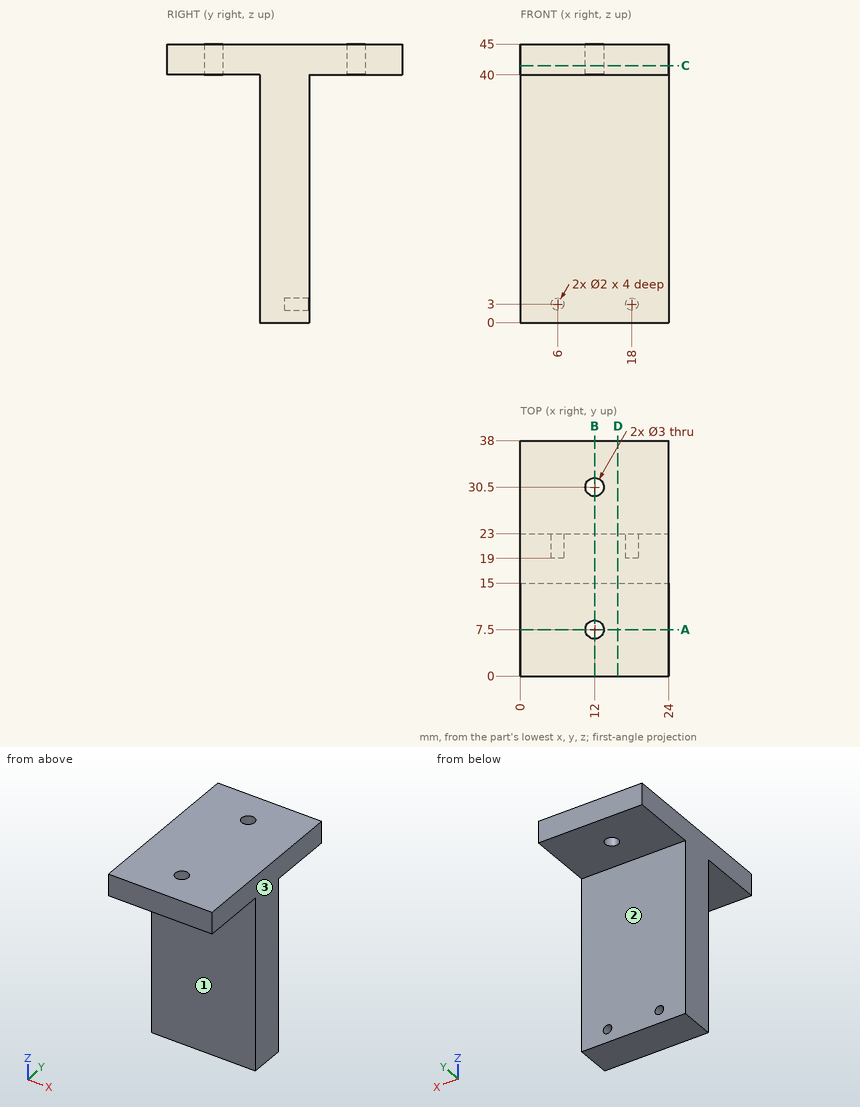
Geometry check sheet. Reference: drawing and pictorial views, mm from the part's lowest x, y, z. A direction names the side the tool comes from. Round coordinates to 2 decimals unless told otherwise and drop trailing zeros. Loops run counter-clockwise (first coordinate to the right, second up) from the corner with the lowest first, then second, coordinate; pieces in that order, holes last. Notation, with made-up numbers: (63, -11.5) - (93, -11.5) arc R20 cw to (93, 4.5) - close; hole circle Ø10 at (55, 19). An arc over 180 degrees is marked (long way). Use a Markdown table: item, result. Add a question column.
1. Access from +Z, -Z, +X, -X, +Y, -Y to the whole of each face (thin tool, end or side, straight path). Record for the marked faces 1, 2 and 3.
2. Section check C-C, the plane z = 41.5. Record the boundary of the cut face in (x, y), plus the area to 3 significant figures.
3. Thickness scan on probe 1 along Y at (x, z) = (12, 43.45); probe 2 along X at (y, z) = (22.05, 3); probe 3 along Z at (x, y) = (6, 21.7). Record the ranges inside material, lowest first. Write a range as [from, to].
4. Gauge pin test, flat ends, axial feed: pin 1 (1 mm diameter, centred on x = 2.5, z = 34, fed in from -Y); pin 2 (1 mm diameter, centred on x = 21, z = 23.5, fed in from +Y); pin 3 (12 mm diameter, centred on x = 13, y = 31.5, fed in from -Z). Record the tip position at first contact, or that the pin passes through.
5. Section check D-D, the plane x = 15.75. Record the boundary of the cut face in (y, z).
6. Section check B-B, the plane x = 12. Record the boundary of the cut face in (y, z), plus the area to 3 significant figures.
7. Section check A-A, the plane y = 7.5. Record the boundary of the cut face in (x, z).
Checks:
| question | item | result |
|---|---|---|
| 1 | face 1 | -Z, +X, -X, -Y |
| 1 | face 2 | -Z, +X, -X, +Y |
| 1 | face 3 | +Z, -Z, +X, +Y, -Y |
| 2 | outline | (0, 0) - (24, 0) - (24, 38) - (0, 38) - close; hole circle Ø3 at (12, 7.5); hole circle Ø3 at (12, 30.5) |
| 2 | area | 898 mm^2 |
| 3 | probe 1 | y = [0, 6], [9, 29], [32, 38] |
| 3 | probe 2 | x = [0, 5], [7, 17], [19, 24] |
| 3 | probe 3 | z = [0, 2], [4, 45] |
| 4 | pin 1 | stops at y = 15 |
| 4 | pin 2 | stops at y = 23 |
| 4 | pin 3 | stops at z = 40 |
| 5 | outline | (0, 40) - (15, 40) - (15, 0) - (23, 0) - (23, 40) - (38, 40) - (38, 45) - (0, 45) - close |
| 6 | outline | (0, 40) - (6, 40) - (6, 45) - (0, 45) - close; (9, 40) - (15, 40) - (15, 0) - (23, 0) - (23, 40) - (29, 40) - (29, 45) - (9, 45) - close; (32, 40) - (38, 40) - (38, 45) - (32, 45) - close |
| 6 | area | 480 mm^2 |
| 7 | outline | (0, 40) - (10.5, 40) - (10.5, 45) - (0, 45) - close; (13.5, 40) - (24, 40) - (24, 45) - (13.5, 45) - close |
